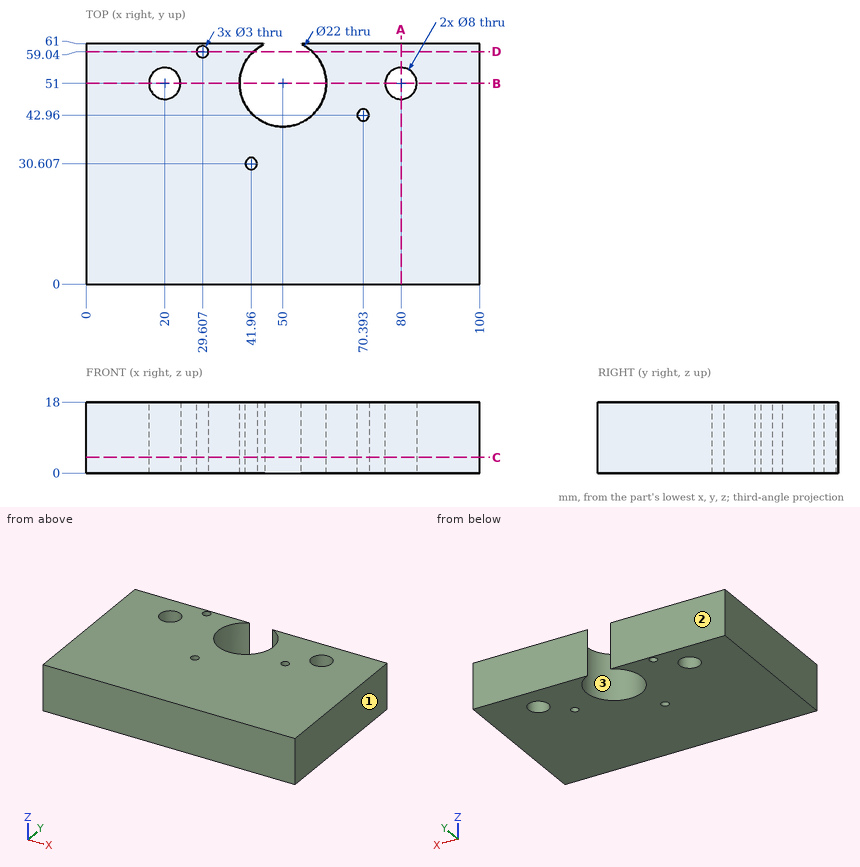
Input: dimensioned drawing with shaded views. Units: mm. Origin: part minimum x, y, z. Round coordinates to 2 decimals unless told otherwise and drop trailing zeros. Loops run counter-clockwise (first coordinate to the right, second up) from the corner with the lowest first, then second, coordinate; pieces in that order, holes last. Notation, with made-up numbers: (-17.75, -35.5) -> (36.25, -35.5) arc R25 cw to (36.25, -13.5) -> close; hole circle Ø7 at (-9.5, -14). An arc over 180 degrees is marked (long way). Answer as a JSON object with one key per item and string values. Group by question number.
Q1. Section query B-B (y = 51). Output: boundary loops of the cut face in (x, z).
Q2. Contact query for flat-ended pins moving along their axis: P1, Ø5, axis at x = 84.5, z = 10, coming from the -Y side; P2, Ø2.5, axis at x = 29.61, y = 59.04, coming from the -Z side. Output: stop coordinate, or through.
Q3. Ray query, line 1 (X direction, y = 41, z = 1.5) (1 decimal); line 2 (X direction, y = 54, z = 1) (1 decimal); line 3 (Y direction, x = 50, z = 4.5). Return the intervals inside material, ascending. Write a range as from..to.
Q4. Section query A-A (x = 80). Output: boundary loops of the cut face in (y, z), plus the area to 3 significant figures.
Q5. Section query C-C (z = 4). Output: boundary loops of the cut face in (x, y), plus the area to 3 significant figures.
Q6. Section query D-D (y = 59.04). Output: boundary loops of the cut face in (x, z).
Q7. Mould query, pull axis Y, two halves, no side actions, for the marked faces 1, 2 and 3. Classes: pulls with the +Y half, pulls with the -Y half, needs draft (parallel to the pull), parting line crosses it, or undercut.
Completed:
{
 "1": {"outline": "(0, 0) -> (16, 0) -> (16, 18) -> (0, 18) -> close; (24, 0) -> (39, 0) -> (39, 18) -> (24, 18) -> close; (61, 0) -> (76, 0) -> (76, 18) -> (61, 18) -> close; (84, 0) -> (100, 0) -> (100, 18) -> (84, 18) -> close"},
 "2": {"P1": "y = 0", "P2": "through"},
 "3": {"line 1": "0..45.4, 54.6..100", "line 2": "0..17.4, 22.6..39.4, 60.6..77.4, 82.6..100", "line 3": "0..40"},
 "4": {"outline": "(0, 0) -> (47, 0) -> (47, 18) -> (0, 18) -> close; (55, 0) -> (61, 0) -> (61, 18) -> (55, 18) -> close", "area": "954 mm²"},
 "5": {"outline": "(0, 0) -> (100, 0) -> (100, 61) -> (54.58, 61) arc R11 cw (long way) to (45.42, 61) -> (0, 61) -> close; hole circle Ø8 at (20, 51); hole circle Ø3 at (29.61, 59.04); hole circle Ø3 at (41.96, 30.61); hole circle Ø3 at (70.39, 42.96); hole circle Ø8 at (80, 51)", "area": "5,600 mm²"},
 "6": {"outline": "(0, 0) -> (28.11, 0) -> (28.11, 18) -> (0, 18) -> close; (31.11, 0) -> (42.49, 0) -> (42.49, 18) -> (31.11, 18) -> close; (57.51, 0) -> (100, 0) -> (100, 18) -> (57.51, 18) -> close"},
 "7": {"face 1": "needs draft", "face 2": "pulls with the +Y half", "face 3": "undercut"}
}
